from build123d import *

# Parameters (mm, degrees)
SKETCH1_W           = 190.5
SKETCH1_H           = 133.35
BOSS_EXTRUDE1_DEPTH = 3.175
SKETCH3_R           = 21.59
CUT_EXTRUDE2_DEPTH  = 117.310785183
SKETCH4_R           = 1.6
SKETCH4_R_2         = 1.599999975
CUT_EXTRUDE3_DEPTH  = 3.175
SKETCH9_R           = 2.5273
CUT_EXTRUDE5_DEPTH  = 10
SKETCH12_W          = 98.425
SKETCH12_H          = 133.35
CUT_EXTRUDE6_DEPTH  = 117.310785183
SKETCH13_R          = 3.175
CUT_EXTRUDE7_DEPTH  = 117.310785183


with BuildPart() as part:
    # Sketch1 → Boss-Extrude1 (new body)
    with BuildSketch(Plane(origin=(0, 0, 0), x_dir=(1, 0, 0), z_dir=(0, 1, 0))):
        Rectangle(SKETCH1_W, SKETCH1_H)
    extrude(amount=BOSS_EXTRUDE1_DEPTH)

    # Sketch3 → Cut-Extrude2 (cut, through all)
    with BuildSketch(Plane(origin=(0, 3.175, 0), x_dir=(1, 0, 0), z_dir=(0, 1, 0))):
        with Locations(Location((-53.425, 0, 0), (0, 0, 270))):
            Circle(SKETCH3_R)
    extrude(amount=-CUT_EXTRUDE2_DEPTH, mode=Mode.SUBTRACT)

    # Sketch4 → Cut-Extrude3 (cut)
    with BuildSketch(Plane(origin=(0, 3.175, 0), x_dir=(1, 0, 0), z_dir=(0, 1, 0))):
        with Locations(Location((-70.425, 17, 0), (0, 0, 270))):
            Circle(SKETCH4_R)
        with Locations(Location((-36.425, 17, 0), (0, 0, 270))):
            Circle(SKETCH4_R_2)
        with Locations(Location((-70.425, -17, 0), (0, 0, 270))):
            Circle(SKETCH4_R)
        with Locations(Location((-36.425, -17, 0), (0, 0, 270))):
            Circle(SKETCH4_R)
    extrude(amount=-CUT_EXTRUDE3_DEPTH, mode=Mode.SUBTRACT)

    # Sketch9 → Cut-Extrude5 (cut)
    with BuildSketch(Plane(origin=(0, 3.175, 0), x_dir=(1, 0, 0), z_dir=(0, 1, 0))):
        with Locations(Location((-18.4365, 0, 0), (0, 0, 270))):
            Circle(SKETCH9_R)
    extrude(amount=-CUT_EXTRUDE5_DEPTH, mode=Mode.SUBTRACT)

    # Sketch12 → Cut-Extrude6 (cut, through all)
    with BuildSketch(Plane(origin=(0, 3.175, 0), x_dir=(1, 0, 0), z_dir=(0, 1, 0))):
        with Locations((46.0375, 0)):
            Rectangle(SKETCH12_W, SKETCH12_H)
    extrude(amount=-CUT_EXTRUDE6_DEPTH, mode=Mode.SUBTRACT)

    # Sketch13 → Cut-Extrude7 (cut, through all)
    with BuildSketch(Plane(origin=(0, 3.175, 0), x_dir=(1, 0, 0), z_dir=(0, 1, 0))):
        with Locations(Location((-63.5, -57.15, 0), (0, 0, 270))):
            Circle(SKETCH13_R)
        with Locations(Location((-31.75, -57.15, 0), (0, 0, 270))):
            Circle(SKETCH13_R)
        with Locations(Location((-85.725, -34.925, 0), (0, 0, 270))):
            Circle(SKETCH13_R)
        with Locations(Location((-85.725, 34.925, 0), (0, 0, 90))):
            Circle(SKETCH13_R)
        with Locations(Location((-31.75, 57.15, 0), (0, 0, 90))):
            Circle(SKETCH13_R)
        with Locations(Location((-63.5, 57.15, 0), (0, 0, 90))):
            Circle(SKETCH13_R)
    extrude(amount=-CUT_EXTRUDE7_DEPTH, mode=Mode.SUBTRACT)


solid = part.part
Geometry: final body of the model. Coordinates: model frame, mm. Round coordinates to 2 decimals unless told otherwise and drop trailing zeros. Order: outer loops, then holes, each group sorted by start corner. A loop starts at its lowest first (then second) coordinate and runs counter-clockwise, first axis right, second up. Notation, with made-up numbers: (4, 28.25) - (16, 28.25) arc R15 cw to (16, 50.25) - close; hole circle Ø2 at (81.25, -1.5). An arc over 180 degrees is marked (long way). Write each question's results on one line, items separated by ' | '.
Item 1: Mould query, pull axis Z, two halves, no side actions, for faces 1 (the cylindrical face through (-29.82, 1.61, -54.63)), 2 (the flat face through (-3.175, 2, 1)), 3 (the flat face through (-50, 2, -66.675)), 4 (the flat face through (-50, 2, 66.675)). Classes: pulls with the +Z half, pulls with the -Z half, needs draft (parallel to the pull), parting line crosses it, or undercut.
Completed:
face 1: undercut | face 2: needs draft | face 3: pulls with the -Z half | face 4: pulls with the +Z half
Item 2: Section B-B, the plane z = -17. Return the cut outline in (x, y) (3 decimals).
Completed:
outline: (-95.25, 0) - (-72.025, 0) - (-72.025, 3.175) - (-95.25, 3.175) - close; (-68.825, 0) - (-66.734, 0) - (-66.734, 3.175) - (-68.825, 3.175) - close; (-40.116, 0) - (-38.025, 0) - (-38.025, 3.175) - (-40.116, 3.175) - close; (-34.825, 0) - (-3.175, 0) - (-3.175, 3.175) - (-34.825, 3.175) - close
Item 3: Material intervals for line 1 along X through (y, z) = (1.7, 57.15) (3 decimals); line 2 along Z through (x, y) = (-65, 0.3) (3 decimals); line 3 along Z through (x, y) = (-84.5, 1.1) (3 decimals), sorted ascending. Write a range as [from, to].
Completed:
line 1: [-95.25, -66.675], [-60.325, -34.925], [-28.575, -3.175] | line 2: [-66.675, -59.948], [-54.352, -18.225], [18.225, 54.352], [59.948, 66.675] | line 3: [-66.675, -37.854], [-31.996, 31.996], [37.854, 66.675]
Item 4: Section A-A, the plane z = 57.15. Return the cut outline in (x, y) (3 decimals).
Completed:
outline: (-95.25, 0) - (-66.675, 0) - (-66.675, 3.175) - (-95.25, 3.175) - close; (-60.325, 0) - (-34.925, 0) - (-34.925, 3.175) - (-60.325, 3.175) - close; (-28.575, 0) - (-3.175, 0) - (-3.175, 3.175) - (-28.575, 3.175) - close
Item 5: Section D-D, the plane y = 1.7. State how many separate pieces and enclosed holes the cut face has, and give its area (3 significant figures).
Completed:
separate pieces: 1 | enclosed holes: 12 | area: 10,600 mm^2
Item 6: Section C-C, the plane x = -49. Return the cut outline in (y, z) (3 decimals).
Completed:
outline: (0, -66.675) - (3.175, -66.675) - (3.175, -21.132) - (0, -21.132) - close; (0, 21.132) - (3.175, 21.132) - (3.175, 66.675) - (0, 66.675) - close
